Part model, mm, in its own coordinate system. Face numbers are marked on the shaded views. Round coordinates to 2 decimals unless told otherwise and drop trailing zeros. Order: outer loops, then holes, each group sorted by start corner. A loop starts at its lowest first (then second) coordinate and runs counter-clockwise, first axis right, second up. Notation, with made-up numbers: (39, 7) - (48, 7) arc R22 ccw to (48, 42) - close; hole circle Ø1 at (56, -20.75). An arc over 180 degrees is marked (long way). Answer as a JSON object with one key per item and string values.
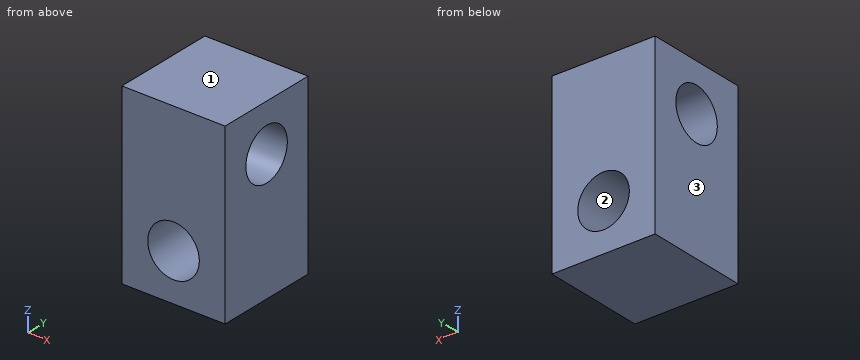
```python
from build123d import *

# Parameters (mm, degrees)
F0_W     = 24
F0_H     = 24
F1_DEPTH = 41
F2_R     = 6
F3_DEPTH = 25
F4_R     = 6
F5_DEPTH = 25


with BuildPart() as f1:
    # F0 (on Top) → F1 (new body)
    with BuildSketch(Plane.XY):
        with Locations((12, 12)):
            Rectangle(F0_W, F0_H)
    extrude(amount=F1_DEPTH)

    # F2 (on face) → F3 (cut)
    with BuildSketch(Plane.XZ):
        with Locations((12, 11)):
            Circle(F2_R)
    extrude(amount=-F3_DEPTH, mode=Mode.SUBTRACT)

    # F4 (on face) → F5 (cut)
    with BuildSketch(Plane(origin=(0, 0, 0), x_dir=(0, -1, 0), z_dir=(-1, 0, 0))):
        with Locations((-12, 30)):
            Circle(F4_R)
    extrude(amount=-F5_DEPTH, mode=Mode.SUBTRACT)


solid = f1.part
```
Item 1: Probe L1, parallel to Z at x = 12, y = 12; L2, parallel to Z at x = 16.75, y = 16.5; L3, parallel to Z at x = 12.25, y = 4.25. List the from-to ranges inside material, lowest first. Write a range as from..to.
Taken from the geometry:
{"L1": "0..5, 17..24, 36..41", "L2": "0..7.33, 14.67..26.03, 33.97..41", "L3": "0..5.01, 16.99..41"}
Item 2: Cut at A-A (x = 12). Write the cut outline in (y, z), plus the area to 3 significant figures.
Taken from the geometry:
{"outline": "(0, 0) - (24, 0) - (24, 5) - (0, 5) - close; (0, 17) - (24, 17) - (24, 41) - (0, 41) - close; hole circle Ø12 at (12, 30)", "area": "583 mm2"}
Item 3: Two-plate mould, pull along Z, no slides. Class the marked faces 1, 2 and 3: pulls with the +Z half, pulls with the -Z half, needs draft (parallel to the pull), parting line crosses it, or undercut.
Taken from the geometry:
{"face 1": "pulls with the +Z half", "face 2": "undercut", "face 3": "needs draft"}
Item 4: Cut at C-C (y = 16.25). Write the cut outline in (x, z), plus the area to 3 significant figures.
Taken from the geometry:
{"outline": "(0, 0) - (24, 0) - (24, 25.76) - (0, 25.76) - close; (0, 34.24) - (24, 34.24) - (24, 41) - (0, 41) - close; hole circle Ø12 at (12, 11)", "area": "668 mm2"}
Item 5: Cut at D-D (x = 4.25). Write the cut outline in (y, z), plus the area to 3 significant figures.
Taken from the geometry:
{"outline": "(0, 0) - (24, 0) - (24, 41) - (0, 41) - close; hole circle Ø12 at (12, 30)", "area": "871 mm2"}
Item 6: Cut at B-B (z = 11). Write the cut outline in (x, y).
Taken from the geometry:
{"outline": "(0, 0) - (6, 0) - (6, 24) - (0, 24) - close; (18, 0) - (24, 0) - (24, 24) - (18, 24) - close"}
